Geometry: final body of the model. Coordinates: model frame, mm. Face numbers are marked on the shaded views. Give positions to 0.01 mm unless a question says otherwise; leave off trailing zeros. Loops run counter-clockwise (first coordinate to the right, second up) from the corner with the lowest first, then second, coordinate; pieces in that order, holes last. Notation, with made-up numbers: (-30.5, 51.25) -> (5.5, 51.25) arc R26 cw to (5.5, 66.25) -> close; hole circle Ø1 at (6, 70). An arc over 180 degrees is marked (long way). Answer in a Markdown table with one row per item. Add a question column.
1) First-contact query: P1, Ø2, axis at y = 4.5, z = 2.5, coming from the -X side. Flat tip, straight axial feed; report the tip coordinate or a pass-through.
2) Draft query along Y for the marked faces 1, 2, 3 and 4. Return one class per face: +Y half, -Y half, draft (parallel to the pull), parting line (faces both ways), or undercut.
3) Section query D-D (y = 4.25). Give the number of separate pieces and of enclosed holes in the cut face, plus the area to 3 significant figures.
4) Section query A-A (x = 16.55). Return the cut outline in (y, z), plus the area to 3 significant figures.
5) Line query: line 1 (Y direction, x = 16.55, z = 0.85); line 2 (X direction, y = 2, z = 0.7); line 3 (X direction, y = 3.25, z = 2.15). Output: solid intervals per line, ascending. Write a range as from..to.
6) Section query B-B (z = 3.35). Return the cut outline in (x, y), plus the area to 3 significant figures.
7) Section query C-C (z = 2.3). Return the cut outline in (x, y).
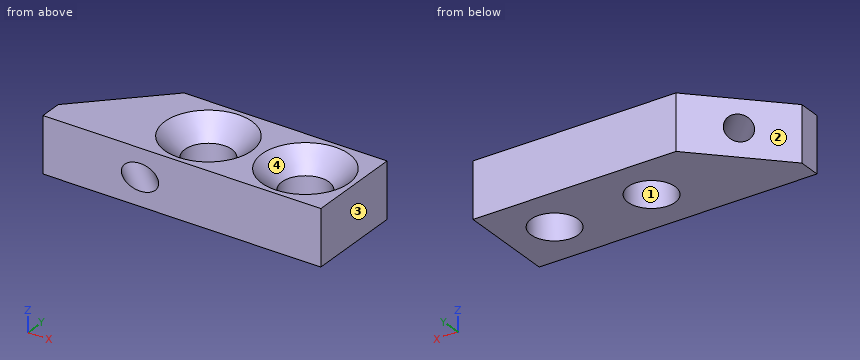
```python
from build123d import *

# Parameters (mm, degrees)
BOSS_EXTRUDE1_DEPTH                                 = 4
CSK_FOR_M3_COUNTERSUNK_FLAT_HEAD_SCREW1_D           = 3.4
CSK_FOR_M3_COUNTERSUNK_FLAT_HEAD_SCREW1_CSINK_D     = 6.3
CSK_FOR_M3_COUNTERSUNK_FLAT_HEAD_SCREW1_CSINK_ANGLE = 90
TAP_DRILL_FOR_M2_TAP1_D                             = 1.9


with BuildPart() as part:
    # Sketch1 → Boss-Extrude1 (new body)
    with BuildSketch(Plane.XY):
        Polygon((5.396358967, 7), (20.05, 7), (20.05, 0), (0, 0), (0, 1.603641033), align=None)
    extrude(amount=BOSS_EXTRUDE1_DEPTH)

    # CSK for M3 Countersunk Flat Head Screw1 (through all)
    with Locations(Plane.XY.offset(4)):
        with Locations((16.55, 3.5), (9.55, 3.5)):
            CounterSinkHole(CSK_FOR_M3_COUNTERSUNK_FLAT_HEAD_SCREW1_D / 2, CSK_FOR_M3_COUNTERSUNK_FLAT_HEAD_SCREW1_CSINK_D / 2, counter_sink_angle=CSK_FOR_M3_COUNTERSUNK_FLAT_HEAD_SCREW1_CSINK_ANGLE)

    # Tap Drill for M2 Tap1 (through all)
    with Locations(Plane(origin=(-0.801820516, 0.801820516, 0), x_dir=(0.7071067811865511, 0.707106781186544, 0), z_dir=(-0.707106781186544, 0.7071067811865511, 0))):
        with Locations((4.949747468, -2)):
            Hole(TAP_DRILL_FOR_M2_TAP1_D / 2)


solid = part.part
```
Evaluation:
| question | item | result |
|---|---|---|
| 1 | P1 | x = 1.9 |
| 2 | face 1 | undercut |
| 2 | face 2 | +Y half |
| 2 | face 3 | draft |
| 2 | face 4 | undercut |
| 3 | separate pieces | 3 |
| 3 | enclosed holes | 0 |
| 3 | area | 38.5 mm² |
| 4 | outline | (0, 0) -> (1.8, 0) -> (1.8, 2.55) -> (0.35, 4) -> (0, 4) -> close; (5.2, 0) -> (7, 0) -> (7, 4) -> (6.65, 4) -> (5.2, 2.55) -> close |
| 4 | area | 12.3 mm² |
| 5 | line 1 | 0..1.8, 5.2..7 |
| 5 | line 2 | 0.4..8.75, 10.35..15.75, 17.35..20.05 |
| 5 | line 3 | 1.65..2.42, 5.08..7.87, 11.23..14.87, 18.23..20.05 |
| 6 | outline | (0, 0) -> (20.05, 0) -> (20.05, 7) -> (5.4, 7) -> (0, 1.6) -> close; hole circle Ø5 at (9.55, 3.5); hole circle Ø5 at (16.55, 3.5) |
| 6 | area | 86.5 mm² |
| 7 | outline | (0, 0) -> (5.73, 0) -> (2.06, 3.66) -> (0, 1.6) -> close; (3.34, 4.94) -> (8.27, 0) -> (20.05, 0) -> (20.05, 7) -> (5.4, 7) -> close; hole circle Ø3.4 at (9.55, 3.5); hole circle Ø3.4 at (16.55, 3.5) |
